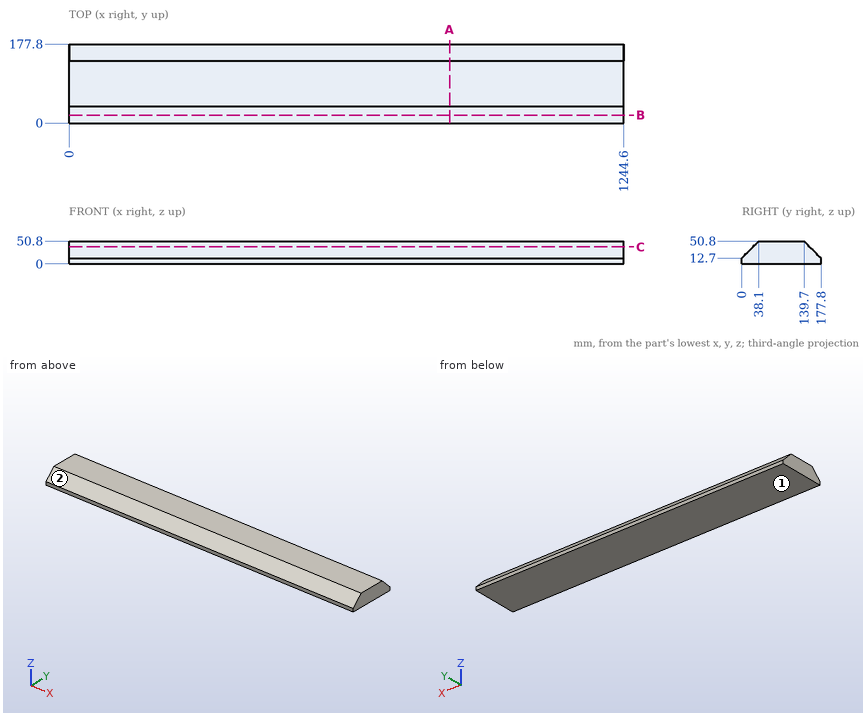
Here's the drawing with two shaded views (mm, measured from the low corner). I have some questions. Give positions to 0.01 mm unless a question says otherwise; leave off trailing zeros. Write each loop counter-clockwise with the first axis right and the second up, starting at its lowest first coordinate (ties: lowest second). Pieces come first, ordered by that corner, then holes. Notation, with made-up numbers: (-37.5, 58) - (-14.5, 58) arc R10 ccw to (-14.5, 69) - close; hole circle Ø2 at (36.25, -9.5). An arc over 180 degrees is marked (long way). Write item = value, one per line. Start each with the question number.
1. Thinking about a two-plate mould opening in Y: for the marked faces 1 and 2, which applies, released by +Y, released by -Y, zero draft, split by the parting line, or undercut?
2. Imagine slicing it at C-C (z = 38). Please give me the cut outline in (x, y).
3. Imagine slicing it at A-A (x = 854). Please give me the cut outline in (y, z), and give its area (3 significant figures).
4. For pin 1 (6 mm diameter, centred on x = 140, z = 31, fed in from -Y); pin 2 (1.5 mm diameter, centred on x = 323.5, y = 37, fed in from +Z); pin 3 (1 mm diameter, centred on x = 172, z = 42.5, fed in from +Y), each with a flat end and sliding along its axis, tell me the tip position at first contact or that it passes through.
5. Please list where these lines run through material, in increasing order: line 1 (Y direction, x = 1184, z = 22); line 2 (Y direction, x = 652, z = 24.5); line 3 (Z direction, x = 851.5, y = 11).
6. Imagine slicing it at B-B (y = 18). Please give me the cut outline in (x, z).
Worked answers:
q1.face_1 = zero draft
q1.face_2 = released by -Y
q2.outline = (0, 25.3) - (1244.6, 25.3) - (1244.6, 152.5) - (0, 152.5) - close
q3.outline = (0, 0) - (177.8, 0) - (177.8, 12.7) - (139.7, 50.8) - (38.1, 50.8) - (0, 12.7) - close
q3.area = 7,580 mm2
q4.pin_1 = 15.3
q4.pin_2 = 50.45
q4.pin_3 = 148.5
q5.line_1 = 9.3 to 168.5
q5.line_2 = 11.8 to 166
q5.line_3 = 0 to 23.7
q6.outline = (0, 0) - (1244.6, 0) - (1244.6, 30.7) - (0, 30.7) - close
